Could you check a few things on this model? Use its own coordinates, in mm. Face numbers are marked on the shaded views. A direction names the side the tool comes from. Coordinates: 2 decimals unless noted, no trailing zeros. Write each loop counter-clockwise with the first axis right and the second up, starting at its lowest first coordinate (ties: lowest second). Pieces come first, ordered by that corner, then holes. Notation, with made-up numbers: M 6,-29 L 38,-29 A23 cw 38,-3 Z; hole C -23.5,39 d9. An arc over 180 degrees is marked long. Write item = value, one per line.
Autodesk Inventor part; units mm, degrees
ref_plane "YZ Plane" through (0, 0, 0) normal (1, 0, 0) x (0, 1, 0)
ref_plane "XZ Plane" through (0, 0, 0) normal (0, 1, 0) x (-1, 0, 0)
ref_plane "XY Plane" through (0, 0, 0) normal (0, 0, 1) x (1, 0, 0)
sketch "Sketch1" plane through (0, 0, 0) normal (0, 1, 0) x (-1, 0, 0)
  line L0 (30, 0) -> (30, -30)
  line L1 (30, -30) -> (0, -30)
  line L2 (0, -30) -> (0, 0)
  arc A0 (15.5, -11.5008) -> (19.5, -11.5008) centre (17.5, -18) ccw
  line L3 (17.5, -18) -> (17.5, -3) construction
  line L4 (15.5, 0) -> (15.5, -11.5008)
  line L5 (19.5, -11.5008) -> (19.5, 0)
  line L6 (0, 0) -> (15.5, 0)
  line L7 (19.5, 0) -> (30, 0)
  dimension "d0" = 30
  dimension "d1" = 30
  dimension "d2" = 13.6
  dimension "d3" = 18
  dimension "d8" = 17.5
  dimension "d9" = 4
  dimension "d10" = 2
extrude "Extrusion1" add sketch "Sketch1" along normal blind 60
sketch "Sketch2" plane through (0, 0, 0) normal (1, 0, 0) x (0, 0, -1)
  line L0 (0, 0) -> (30, 0)
  line L1 (30, 0) -> (30, 60)
  line L2 (0, 60) -> (30, 60)
  line L3 (0, 0) -> (0, 60)
  line L4 (11.5008, 0) -> (11.5008, 60)
  circle A0 centre (6, 30) radius 3
  dimension "d14" = 6
  dimension "d15" = 30
  dimension "d16" = 6
extrude "Extrusion2" cut sketch "Sketch2" against normal through all contours A0
sketch "Sketch3" plane through (-30, 0, -30) normal (-1, 0, 0) x (0, 0, 1)
  line L0 (30, 0) -> (30, 60)
  circle A0 centre (24, 30) radius 3 construction
  line L1 (19.7, 27.5174) -> (19.7, 32.4826)
  line L2 (19.7, 32.4826) -> (24, 34.9652)
  line L3 (24, 34.9652) -> (28.3, 32.4826)
  line L4 (28.3, 32.4826) -> (28.3, 27.5174)
  line L5 (28.3, 27.5174) -> (24, 25.0348)
  line L6 (24, 25.0348) -> (19.7, 27.5174)
  dimension "d31" = 4.3
sketch "Sketch4" plane through (0, 0, 0) normal (1, 0, 0) x (0, 0, -1)
  circle A0 centre (6, 30) radius 3 construction
  line L0 (0, 0) -> (30, 0) construction
  line L1 (30, 0) -> (30, 60) construction
  line L2 (0, 60) -> (30, 60) construction
  line L3 (0, 0) -> (0, 60) construction
  line L4 (30, 60) -> (0, 60) construction
  line L5 (15, 60) -> (15, 0) construction
  line L6 (30, 0) -> (0, 0) construction
  line L7 (0, 0) -> (0, 60) construction
  line L8 (0, 30) -> (30, 30) construction
  circle A1 centre (15, 45) radius 3
  circle A2 centre (15, 15) radius 3
  dimension "d22" = 6
  dimension "d23" = 15
  dimension "d24" = 6
  dimension "d25" = 15
extrude "Extrusion4" cut sketch "Sketch4" against normal blind 10
extrude "Extrusion6" cut sketch "Sketch3" against normal blind 4
sketch "Sketch6" plane through (0, 0, 0) normal (1, 0, 0) x (0, 0, -1)
  circle A0 centre (15, 45) radius 3 construction
  circle A1 centre (15, 15) radius 3 construction
  circle A2 centre (6, 30) radius 3 construction
  line L0 (0, 0) -> (30, 0) construction
  line L1 (30, 0) -> (30, 60) construction
  line L2 (0, 60) -> (30, 60) construction
  line L3 (0, 0) -> (0, 60) construction
  line L4 (30, 0) -> (30, 60) construction
  line L5 (30, 15) -> (0, 15) construction
  line L6 (30, 45) -> (0, 45) construction
  line L7 (0, 0) -> (0, 60) construction
  circle A3 centre (9, 15) radius 1.5
  circle A4 centre (21, 15) radius 1.5
  circle A5 centre (9, 45) radius 1.5
  circle A6 centre (21, 45) radius 1.5
  dimension "d34" = 3
  dimension "d35" = 3
  dimension "d36" = 3
  dimension "d37" = 3
  dimension "d38" = 6
  dimension "d39" = 6
  dimension "d40" = 6
  dimension "d41" = 6
  dimension "d42" = 15
  dimension "d43" = 15
extrude "Extrusion7" add sketch "Sketch6" along normal blind 3.5
sketch "Sketch7" plane through (0, 60, 0) normal (0, 1, 0) x (1, 0, 0)
  circle A0 centre (-5.5, 24.5) radius 3
  line L0 (0, 30) -> (-30, 30)
  line L1 (0, 0) -> (0, 30)
  dimension "d46" = 6
  dimension "d47" = 5.5
  dimension "d48" = 5.5
extrude "Extrusion8" cut sketch "Sketch7" against normal blind 15
properties part number "SupportV2_P1_ComFuros" material "PET Plastic"
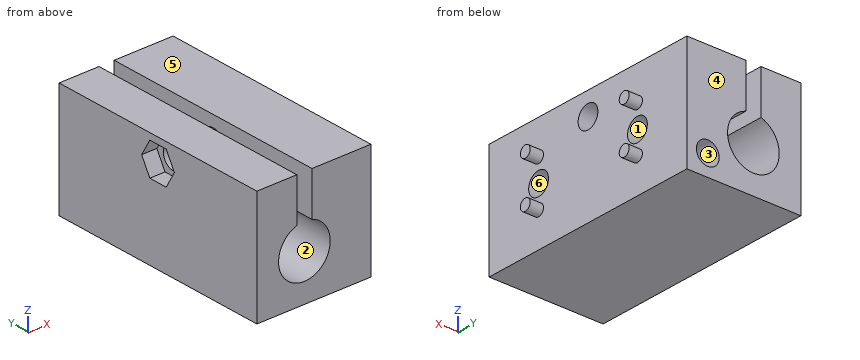
Item 1: If I drill on line 1 along X through (y, z) = (13, -18); line 2 along X through (y, z) = (5, -5); line 3 along Y through (x, z) = (-5.5, -6), over which ranges is the centre line in solid material (lowest first)?
Numbers:
line_1 = -30 to -24.3, -10.7 to 0
line_2 = -30 to -19.5, -15.5 to 0
line_3 = 0 to 27, 33 to 60
Item 2: Imagine slicing it at B-B (z = -23.75). Write out the boundary of the cut face in (x, y).
Numbers:
outline = M -30,0 L -21.13,0 L -21.13,60 L -30,60 Z; M -13.87,0 L 0,0 L 0,60 L -2.6,60 L -2.6,45 L -8.4,45 L -8.4,60 L -13.87,60 Z
Item 3: Imagine slicing it at C-C (y = 15). Write out the boundary of the cut face in (x, z), and give its area (3 significant figures).
Numbers:
outline = M -30,-30 L 0,-30 L 0,-22.5 L 3.5,-22.5 L 3.5,-19.5 L 0,-19.5 L 0,-18 L -10,-18 L -10,-12 L 0,-12 L 0,-10.5 L 3.5,-10.5 L 3.5,-7.5 L 0,-7.5 L 0,0 L -15.5,0 L -15.5,-11.5 A6.8 cw long -19.5,-11.5 L -19.5,0 L -30,0 Z
area = 671 mm²
Item 4: Imagine slicing it at D-D (x = -4.5). Write out the boundary of the cut face in (y, z), and give its area (3 significant figures).
Numbers:
outline = M 0,-30 L 60,-30 L 60,-27.33 L 45,-27.33 L 45,-21.67 L 60,-21.67 L 60,0 L 0,0 Z; hole C 15,-15 d6; hole C 30,-6 d6; hole C 45,-15 d6
area = 1,630 mm²
Item 5: I'm going to push flat-ended pins straight in: P1, Ø5, axis at x = -22.5, z = -17, coming from the -Y side; P2, Ø12.5, axis at y = 28.5, z = -8, coming from the +X side; P3, Ø3, axis at y = 45, z = -16, coming from the +X side; P4, Ø5.5, axis at x = -5.5, z = -24.5, coming from the +Y side. Where does each tip first touch, or does it pass through?
Numbers:
P1 = 0
P2 = 0
P3 = -10
P4 = 45
Item 6: If we mould it in two halves opening along Z, with no side actions, what happens to the marked faces 4, 5 and 6? For each: pulls with the +Z half, pulls with the -Z half, needs draft (parallel to the pull), parting line crosses it, or undercut.
Numbers:
face_4 = needs draft
face_5 = pulls with the +Z half
face_6 = undercut
Item 7: Imagine slicing it at A-A (y = 29). Write out the boundary of the cut face in (x, z), and give its area (3 significant figures).
Numbers:
outline = M -30,-30 L 0,-30 L 0,-8.83 L -15.5,-8.83 L -15.5,-11.5 A6.8 cw long -19.5,-11.5 L -19.5,-8.83 L -26,-8.83 L -26,-10.3 L -30,-10.3 Z; M -30,-1.7 L -26,-1.7 L -26,-3.17 L -19.5,-3.17 L -19.5,0 L -30,0 Z; M -15.5,-3.17 L 0,-3.17 L 0,0 L -15.5,0 Z
area = 551 mm²
Item 8: For the marked faces 1, 2 and 3, which set-ups out of +Z, -Z, +X, -X, +Y, -Y let a thin tool reach every point of the face, with its end or its side?
Numbers:
face_1 = +X
face_2 = +Y, -Y
face_3 = +Y
